Autodesk Inventor part; units mm, degrees
ref_plane "YZ Plane" through (0, 0, 0) normal (1, 0, 0) x (0, 1, 0)
ref_plane "XZ Plane" through (0, 0, 0) normal (0, 1, 0) x (-1, 0, 0)
ref_plane "XY Plane" through (0, 0, 0) normal (0, 0, 1) x (1, 0, 0)
sketch "Skizze5" plane through (0, 0, 0) normal (0, 0, 1) x (1, 0, 0)
  line L0 (-257.6, 0) -> (257.6, 0)
  line L1 (0, -257.6) -> (0, 257.6)
  circle A0 centre (0, 0) radius 184
  line L2 (0, 0) -> (0, 184)
  line L3 (-7.5, 183.8471) -> (7.5, 183.8471)
  line L4 (-7.5, 183.8471) -> (-7.5, 163.8471)
  line L5 (7.5, 183.8471) -> (7.5, 163.8471)
  line L6 (-7.5, 163.8471) -> (7.5, 163.8471)
  dimension "d14" = 368
  dimension "d15" = 15
  dimension "d16" = 20
  dimension "d17" = 20
extrude "Extrusion3" add sketch "Skizze5" along normal blind 3 contours L6 L4 L3 L1 | L1 L3 L5 L6 | L3 L1 A0 | A0 L1 L3
sketch "Skizze6" plane through (0, 0, 0) normal (0, 0, -1) x (-1, 0, 0)
  line L0 (-7.5, 163.8471) -> (-7.5, 183.8471)
  arc A0 (7.5, 183.8471) -> (-7.5, 183.8471) centre (0, 0) ccw
  arc A1 (-7.5, 183.8471) -> (0, 184) centre (0, 0) ccw
  line L1 (-7.5, 183.8471) -> (7.5, 183.8471)
  line L2 (7.5, 183.8471) -> (7.5, 180.8471)
  line L3 (7.5, 180.8471) -> (-7.5, 180.8471)
  line L4 (-7.5, 180.8471) -> (-7.5, 183.8471)
  point P0 (7.5, 183.8471)
  point P1 (-7.5, 180.8471)
  dimension "d20" = 3
extrude "Extrusion4" add sketch "Skizze6" along normal blind 17 contours L0 L1 L2 L3 | A0 L1
sketch "Skizze7" plane through (0, 0, 3) normal (0, 0, 1) x (1, 0, 0)
  line L0 (-7.5, 163.8471) -> (7.5, 163.8471)
  circle A0 centre (0, 168.8471) radius 2.5
  point P0 (0, 0)
  dimension "d23" = 5
  dimension "d24" = 5
extrude "Extrusion5" cut sketch "Skizze7" against normal blind 17
properties part number "WinkelVentilator"
For this review, take the finished solid that the model builds, in its own axes (mm). A direction names the side the tool comes from. Round coordinates to 2 decimals unless told otherwise and drop trailing zeros. Write each loop counter-clockwise with the first axis right and the second up, starting at its lowest first coordinate (ties: lowest second). Pieces come first, ordered by that corner, then holes. Notation, with made-up numbers: (2.5, 17) - (50.5, 17) arc R37 ccw to (50.5, 55) - close; hole circle Ø7 at (-16.5, 78.25). An arc over 180 degrees is marked (long way). Put each result on its own line as item: value.
Q1. Insertion check: pin 1 Ø2 at (x, z) = (-5, -14.5) entering from +Y; pin 2 Ø6 at (x, y) = (0, 168.85) entering from -Z; pin 3 Ø3 at (y, z) = (175.5, -2.5) entering from +X. Each pin has a flat end and moves straight along its axis. Give the tip position at first contact, or say it passes through.
Solved:
pin 1: stops at y = 183.96
pin 2: stops at z = 0
pin 3: passes through
Q2. We need section D-D (z = -2). Give the boundary of the cut face in (x, y).
Solved:
outline: (-7.5, 180.85) - (7.5, 180.85) - (7.5, 183.85) arc R184 ccw to (-7.5, 183.85) - close
Q3. Mouldability with a two-part tool opening along X and no side actions: class faces 3 (the face through (1.154, 166.629, 1.521)), 4 (the face through (0, 180.847, -8)), 5 (the face through (-7.5, 181, -3)) as released by +X, released by -X, zero draft, split by the parting line, or undercut.
Solved:
face 3: undercut
face 4: zero draft
face 5: released by -X
Q4. We need section C-C (z = 1). Give the boundary of the cut face in (x, y).
Solved:
outline: (-7.5, 163.85) - (7.5, 163.85) - (7.5, 183.85) arc R184 ccw to (-7.5, 183.85) - close; hole circle Ø5 at (0, 168.85)
Q5. Machinability: for faces 1 (the face through (0, 182, -17)), 2 (the face through (0, 172, 0)), which of the approach directions +Z, -Z, +X, -X, +Y, -Y give a long, thin tool a straight path to every point of the face, cutting with its end or side? Answer none if there is none.
Solved:
face 1: -Z, +X, -X, +Y, -Y
face 2: -Z, +X, -X, -Y
Q6. We need section A-A (x = 0). Give the boundary of the cut face in (y, z), and give its area (3 significant figures).
Solved:
outline: (163.85, 0) - (166.35, 0) - (166.35, 3) - (163.85, 3) - close; (171.35, 0) - (180.85, 0) - (180.85, -17) - (184, -17) - (184, 3) - (171.35, 3) - close
area: 99.1 mm2
Q7. We need section B-B (y = 168.25). Give the boundary of the cut face in (x, z), and give its area (3 significant figures).
Solved:
outline: (-7.5, 0) - (-2.43, 0) - (-2.43, 3) - (-7.5, 3) - close; (2.43, 0) - (7.5, 0) - (7.5, 3) - (2.43, 3) - close
area: 30.4 mm2
Q8. Wall thickness on probe 1 along Y at (x, z) = (0, 0.8); probe 2 along Z at (x, y) = (-1, 175.5); probe 3 along Y at (x, z) = (1, -12.5): over which ranges is each line inside the solid? List them lowest first.
Solved:
probe 1: y = 163.85 to 166.35, 171.35 to 184
probe 2: z = 0 to 3
probe 3: y = 180.85 to 184
